Autodesk Fusion 360 part; units mm, degrees
sketch "Sketch1" plane through (0, 0, 0) normal (1, 0, 0) x (0, 1, 0)
sketch "Sketch2" plane through (0, 0, 0) normal (0, 0, 1) x (1, 0, 0)
  circle A0 centre (0, 0) radius 15
  dimension "d1" = 30
extrude "Extrude1" add sketch "Sketch2" along normal blind 135
sketch "Sketch3" plane through (0, 0, 135) normal (0, 0, 1) x (-1, 0, 0)
  circle A0 centre (0, 0) radius 15
  line L0 (9, 9) -> (-9, 9)
  line L1 (-9, 9) -> (-9, -9)
  line L2 (-9, -9) -> (9, -9)
  line L3 (9, -9) -> (9, 9)
  line L4 (9, 9) -> (-9, -9) construction
  line L5 (-9, 9) -> (9, -9) construction
  dimension "d4" = 18
  dimension "d5" = 18
extrude "Extrude2" add sketch "Sketch3" along normal blind 10 contours L0 L1 L2 L3
fillet "Fillet1" radius 5 1 edges at (-13.9849, -5.4242, 0)
delete_face "DeleteFace1" 1 faces at (14.8356, -1.4845, 4.0537)
The listing builds one solid part. Answer for the finished solid, in the listing's coordinates (mm). A direction names the side the tool comes from. Give positions to 0.01 mm unless a question says otherwise; leave off trailing zeros. Write each loop counter-clockwise with the first axis right and the second up, starting at its lowest first coordinate (ties: lowest second). Pieces come first, ordered by that corner, then holes. Notation, with made-up numbers: (39, 15) - (76, 15) arc R30 cw to (76, 49) - close; hole circle Ø11 at (-27, 83). An arc over 180 degrees is marked (long way). Use one line per item in the form item = value. Start each with the question number.
1) Find section D-D on y = 13.25. Determine the outline of the cut face in (x, z).
2) A tool of negligible diameter and unlimited length cuts with its end or side. For faces 1 (the face through (-9, 0, 140)), 2 (the face through (0, 9, 140)), 3 (the face through (9, 0, 140)), from which of +Z, -Z, +X, -X, +Y, -Y can it reach the whole face along a straight path? Write none if from no direction.
3) Find section C-C on z = 51. Determine the outline of the cut face in (x, y).
4) Find section A-A on y = 0. Determine the outline of the cut face in (x, z), plus the area to 3 significant figures.
5) Flat-ended cylindrical pins translate along their axes: pin 1 Ø2 at (y, z) = (9, 89) entering from +X; pin 2 Ø11 at (x, z) = (3.5, 142.5) entering from -Y; pin 3 Ø3 at (x, z) = (6.5, 112) entering from +Y. Find the tip coordinate at first contact, or state that the pin passes through.
6) Consider line 1 along Z through (x, y) = (5.75, 10); line 2 along X through (y, z) = (-11.5, 6); line 3 along Y through (x, z) = (-11, 82). Determine where each line is inside the solid, lowest interval first. Write a range as from..to.
Geometry results:
q1.outline = (-7.03, 0) - (7.03, 0) - (7.03, 135) - (-7.03, 135) - close
q2.face_1 = +Z, -X, +Y, -Y
q2.face_2 = +Z, +X, -X, +Y
q2.face_3 = +Z, +X, +Y, -Y
q3.outline = circle Ø30 at (0, 0)
q4.outline = (-15, 0) - (15, 0) - (15, 135) - (9, 135) - (9, 145) - (-9, 145) - (-9, 135) - (-15, 135) - close
q4.area = 4,230 mm2
q5.pin_1 = 12.69
q5.pin_2 = -9
q5.pin_3 = 14.14
q6.line_1 = 0..135
q6.line_2 = -9.63..9.63
q6.line_3 = -10.2..10.2
